Work out the finished part from the listing and answer in its coordinate system (mm). A direction names the side the tool comes from. Give positions to 0.01 mm unless a question says otherwise; leave off trailing zeros. Loops run counter-clockwise (first coordinate to the right, second up) from the corner with the lowest first, then second, coordinate; pieces in that order, holes last. Notation, with made-up numbers: (32.25, -28) - (84.25, -28) arc R26 cw to (84.25, 0) - close; hole circle Ø5 at (24, 87.25). An arc over 180 degrees is marked (long way). One line per question, with ' | ' between items.
Autodesk Inventor part; units mm, degrees
ref_plane "작업 평면1" through (0, 2.5, 0) normal (0, 1, 0) x (1, 0, 0)
ref_plane "YZ Plane" through (0, 0, 0) normal (1, 0, 0) x (0, 1, 0)
ref_plane "XZ Plane" through (0, 0, 0) normal (0, 1, 0) x (-1, 0, 0)
sketch "스케치1" plane through (0, 0, 0) normal (0, 1, 0) x (-1, 0, 0)
  line L0 (-32.4, -32.4) -> (32.4, -32.4)
  line L1 (32.4, -32.4) -> (32.4, 32.4)
  line L2 (32.4, 32.4) -> (-32.4, 32.4)
  line L3 (-32.4, 32.4) -> (-32.4, -32.4)
  line L4 (-32.4, -32.4) -> (32.4, 32.4) construction
  line L5 (32.4, -32.4) -> (-32.4, 32.4) construction
  line L6 (-30, 30) -> (30, 30)
  line L7 (30, 30) -> (30, -30)
  line L8 (30, -30) -> (-30, -30)
  line L9 (-30, -30) -> (-30, 30)
  line L10 (-30, 30) -> (30, -30) construction
  line L11 (30, 30) -> (-30, -30) construction
  point P0 (0, 0)
  dimension "d13" = 60
  dimension "d14" = 60
  dimension "d15" = 2.4
  dimension "d16" = 2.4
extrude "돌출1" add sketch "스케치1" along normal blind 5 contours L3 L2 L1 L0 | L6 L7 L8 L9
sketch "스케치2" plane through (0, 5, 0) normal (0, 1, 0) x (1, 0, 0)
  line L0 (30, 30) -> (-30, 30)
  line L1 (-30, 30) -> (-30, -30)
  line L2 (-30, -30) -> (30, -30)
  line L3 (30, -30) -> (30, 30)
  line L4 (30, 30) -> (-30, -30) construction
  line L5 (-30, 30) -> (30, -30) construction
  line L6 (31.6, -31.6) -> (-31.6, -31.6)
  line L7 (-31.6, -31.6) -> (-31.6, 31.6)
  line L8 (-31.6, 31.6) -> (31.6, 31.6)
  line L9 (31.6, 31.6) -> (31.6, -31.6)
  line L10 (31.6, -31.6) -> (-31.6, 31.6) construction
  line L11 (-31.6, -31.6) -> (31.6, 31.6) construction
  point P0 (0, 0)
  dimension "d4" = 60
  dimension "d5" = 60
  dimension "d6" = 1.6
extrude "돌출2" cut sketch "스케치2" against normal blind 1.6
sketch "스케치3" plane through (0, 5, 0) normal (0, 1, 0) x (1, 0, 0)
  line L0 (26.25, -26.25) -> (-26.25, -26.25)
  line L1 (-26.25, -26.25) -> (-26.25, 26.25)
  line L2 (-26.25, 26.25) -> (26.25, 26.25)
  line L3 (26.25, 26.25) -> (26.25, -26.25)
  line L4 (26.25, -26.25) -> (-26.25, 26.25) construction
  line L5 (-26.25, -26.25) -> (26.25, 26.25) construction
  point P0 (0, 0)
  dimension "d9" = 52.5
  dimension "d10" = 52.5
extrude "돌출3" cut sketch "스케치3" against normal blind 5
ref_plane "작업 평면1" through (0, 2.5, 0) normal (0, 1, 0) x (1, 0, 0)
mirror "미러1" about plane through (0, 2.5, 0) normal (0, 1, 0) of "돌출2"
properties part number "사각형 OV-PAM 5패턴 링"
1. Consider L1, parallel to Z at x = 15, y = 3.65; L2, parallel to Z at x = 14, y = 1.9. Determine where each line is inside the solid, lowest interval first.
Evaluation:
L1: -32.4 to -31.6, -30 to -26.25, 26.25 to 30, 31.6 to 32.4 | L2: -32.4 to -26.25, 26.25 to 32.4
2. Find section C-C on y = 2.65. Write down the section's boundary in (x, z).
Evaluation:
outline: (-32.4, -32.4) - (32.4, -32.4) - (32.4, 32.4) - (-32.4, 32.4) - close; hole (-26.25, -26.25) - (26.25, -26.25) - (26.25, 26.25) - (-26.25, 26.25) - close
3. Find section A-A on z = -2. Write down the section's boundary in (x, y), then the cut area to 3 significant figures.
Evaluation:
outline: (-32.4, 0) - (-31.6, 0) - (-31.6, 1.6) - (-30, 1.6) - (-30, 0) - (-26.25, 0) - (-26.25, 5) - (-30, 5) - (-30, 3.4) - (-31.6, 3.4) - (-31.6, 5) - (-32.4, 5) - close; (26.25, 0) - (30, 0) - (30, 1.6) - (31.6, 1.6) - (31.6, 0) - (32.4, 0) - (32.4, 5) - (31.6, 5) - (31.6, 3.4) - (30, 3.4) - (30, 5) - (26.25, 5) - close | area: 51.3 mm2
4. Determine the mould class of faces 1 (the flat face through (32.4, 2, 0)), 2 (the flat face through (0, 2, -32.4)), 3 (the flat face through (0, 1, 30)) for opening direction X: +X half, -X half, draft (parallel to the pull), parting line (faces both ways), or undercut.
Evaluation:
face 1: +X half | face 2: draft | face 3: undercut
5. Find section D-D on z = 28. Write down the section's boundary in (x, y), then the cut area to 3 significant figures.
Evaluation:
outline: (-32.4, 0) - (-31.6, 0) - (-31.6, 1.6) - (-30, 1.6) - (-30, 0) - (30, 0) - (30, 1.6) - (31.6, 1.6) - (31.6, 0) - (32.4, 0) - (32.4, 5) - (31.6, 5) - (31.6, 3.4) - (30, 3.4) - (30, 5) - (-30, 5) - (-30, 3.4) - (-31.6, 3.4) - (-31.6, 5) - (-32.4, 5) - close | area: 314 mm2
6. Find section B-B on x = -8.5. Write down the section's boundary in (y, z).
Evaluation:
outline: (0, -32.4) - (5, -32.4) - (5, -31.6) - (3.4, -31.6) - (3.4, -30) - (5, -30) - (5, -26.25) - (0, -26.25) - (0, -30) - (1.6, -30) - (1.6, -31.6) - (0, -31.6) - close; (0, 26.25) - (5, 26.25) - (5, 30) - (3.4, 30) - (3.4, 31.6) - (5, 31.6) - (5, 32.4) - (0, 32.4) - (0, 31.6) - (1.6, 31.6) - (1.6, 30) - (0, 30) - close
7. A flat-ended cylindrical pin translates along its axis: pin 1 (12 mm diameter, centred on x = -5, z = 22.5, fed in from +Y). Find the tip coordinate at first contact, or state that the pin passes through.
Evaluation:
pin 1: y = 5
8. Which of the six approach directions +Z, -Z, +X, -X, +Y, -Y give full straight-line access (tool end or side, diameter ignored) to faces 4 (the flat face through (-31.6, 4, 0)), 5 (the flat face through (-32.4, 2, 0)), 6 (the flat face through (0, 1, -30))?
Evaluation:
face 4: +Y | face 5: +Z, -Z, -X, +Y, -Y | face 6: -Y
